Print and shaded views of the part. All mm, measured from the part's lowest x, y and z. A direction names the side the tool comes from. Round coordinates to 2 decimals unless told otherwise and drop trailing zeros. Loops run counter-clockwise (first coordinate to the right, second up) from the corner with the lowest first, then second, coordinate; pieces in that order, holes last. Notation, with made-up numbers: (-15.75, -27.5) - (21.25, -27.5) arc R24 cw to (21.25, -0.5) - close; hole circle Ø10 at (39.5, 60.25). An arc over 180 degrees is marked (long way). Answer as a JSON object with one key per item and string values.
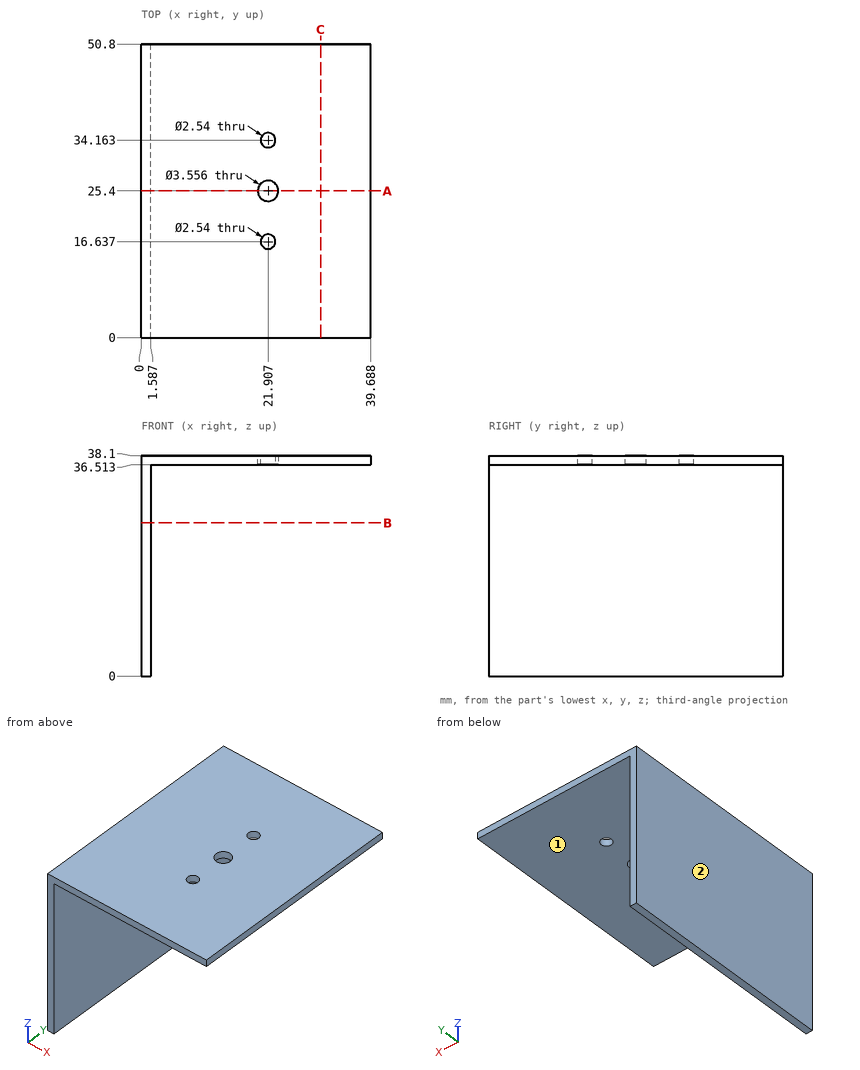
1) Slice it at A-A on y = 25.4. List the corners of the cut face in (x, z) (1 decimal), then the cut area to 3 significant figures.
Values follow:
{"outline": "(0, 0) - (1.6, 0) - (1.6, 36.5) - (20.1, 36.5) - (20.1, 38.1) - (0, 38.1) - close; (23.7, 36.5) - (39.7, 36.5) - (39.7, 38.1) - (23.7, 38.1) - close", "area": "115 mm²"}
2) Drop flat-ended pins along their axis: P1, Ø4, axis at x = 18, y = 9.5, coming from the -Z side; P2, Ø4, axis at x = 21.91, y = 16.64, coming from the +Z side; P3, Ø10, axis at y = 41, z = 18.5, coming from the +X side; P4, Ø3, axis at x = 21.91, y = 25.4, coming from the +Z side. Give the stop position or say it passes through.
Values follow:
{"P1": "z = 36.51", "P2": "z = 38.1", "P3": "x = 1.59", "P4": "through"}
3) Probe probe 1 along Z at (x, y) = (27, 16.5); probe 2 along X at (y, z) = (46.5, 2.5). List the from-to ranges inside material, lowest first.
Values follow:
{"probe 1": "36.51 to 38.1", "probe 2": "0 to 1.59"}
4) Slice it at B-B on z = 26.5. List the corners of the cut face in (x, y).
Values follow:
{"outline": "(0, 0) - (1.59, 0) - (1.59, 50.8) - (0, 50.8) - close"}
5) Tool access for the marked faces 1 and 2: list every direction of +Z, -Z, +X, -X, +Y, -Y with a clear straight run to the whole face (end or side of a thin tool).
Values follow:
{"face 1": "-Z, +X, +Y, -Y", "face 2": "+Z, -Z, -X, +Y, -Y"}
6) Slice it at C-C on x = 31. List the corners of the cut face in (y, z).
Values follow:
{"outline": "(0, 36.51) - (50.8, 36.51) - (50.8, 38.1) - (0, 38.1) - close"}
